Geometry check sheet. Reference: the model listing, model coordinates, mm. A direction names the side the tool comes from. Round coordinates to 2 decimals unless told otherwise and drop trailing zeros. Write each loop counter-clockwise with the first axis right and the second up, starting at its lowest first coordinate (ties: lowest second). Pieces come first, ordered by that corner, then holes. Notation, with made-up numbers: M 70,71.25 L 128,71.25 A31 ccw 128,100.25 Z; hole C 73,16.25 d2. An arc over 180 degrees is marked long. Use a Markdown table: item, result.
```python
from build123d import *

# Parameters (mm, degrees)
F0_W     = 343.231324
F0_H     = 343.231324
F1_DEPTH = 12.7


with BuildPart() as f1:
    # F0 (on Front) → F1 (new body)
    with BuildSketch(Plane.XZ):
        Rectangle(F0_W, F0_H)
        with BuildLine():
            ThreePointArc((-114.373991, 87.598695), (-86.679587, 115.357074), (-57.301, 89.38774))
            Line((-57.301, 89.38774), (-57.223991, -84.985509))
            ThreePointArc((-57.223991, -84.985509), (-84.931642, -113.586746), (-114.373991, -86.774572))
            ThreePointArc((-114.373991, -86.774572), (-114.429209, -84.998141), (-114.373991, -83.22171))
            Line((-114.373991, -83.22171), (-114.373991, 85.938318))
            ThreePointArc((-114.373991, 85.938318), (-114.386042, 86.768506), (-114.373991, 87.598695))
        make_face(mode=Mode.SUBTRACT)
        with BuildLine():
            ThreePointArc((114.411461, 86.554876), (114.417905, 85.362723), (114.374665, 84.171337))
            Line((114.374665, 84.171337), (111.931052, -74.1199))
            ThreePointArc((111.931052, -74.1199), (114.392674, -86.177603), (111.560034, -98.153576))
            ThreePointArc((111.560034, -98.153576), (80.104585, -113.767264), (57.224665, -87.126286))
            ThreePointArc((57.224665, -87.126286), (57.190861, -85.736104), (57.224665, -84.345923))
            Line((57.224665, -84.345923), (57.224665, 85.103969))
            ThreePointArc((57.224665, 85.103969), (57.216092, 85.804222), (57.224665, 86.504474))
            ThreePointArc((57.224665, 86.504474), (85.793493, 114.406821), (114.411461, 86.554876))
        make_face(mode=Mode.SUBTRACT)
    extrude(amount=F1_DEPTH)


solid = f1.part
```
Item 1: Cross-section at A-A, the plane y = -10.5. Record the cut outline in (x, z).
Outcome:
| item | result |
|---|---|
| outline | M -171.62,-171.62 L 171.62,-171.62 L 171.62,171.62 L -171.62,171.62 Z; hole M -114.37,-86.77 A28.6 ccw -57.22,-84.99 L -57.3,89.39 A28.6 ccw -114.37,87.6 A28.6 ccw -114.37,85.94 L -114.37,-83.22 A28.6 ccw Z; hole M 57.22,-87.13 A28.6 ccw 111.56,-98.15 A28.6 ccw 111.93,-74.12 L 114.37,84.17 A28.6 ccw 114.41,86.55 A28.6 ccw 57.22,86.5 A28.6 ccw 57.22,85.1 L 57.22,-84.35 A28.6 ccw Z |
Item 2: Cross-section at D-D, the plane z = -107. Record the cut outline in (x, y), and give its area (3 significant figures).
Outcome:
| item | result |
|---|---|
| outline | M -171.62,-12.7 L -104.1,-12.7 L -104.1,0 L -171.62,0 Z; M -67.55,-12.7 L 66.66,-12.7 L 66.66,0 L -67.55,0 Z; M 104.92,-12.7 L 171.62,-12.7 L 171.62,0 L 104.92,0 Z |
| area | 3,410 mm2 |
Item 3: Access from +Z, -Z, +X, -X, +Y, -Y to the whole of each face (thin tool, end or side, straight path). Record for faces 1 (the face through (-2, -6, -171.616)), 2 (the face through (-114.374, -6, 0)).
Outcome:
| item | result |
|---|---|
| face 1 | -Z, +X, -X, +Y, -Y |
| face 2 | +Y, -Y |
Item 4: Cross-section at C-C, the plane z = 34.5. Record the cut outline in (x, y).
Outcome:
| item | result |
|---|---|
| outline | M -171.62,-12.7 L -114.37,-12.7 L -114.37,0 L -171.62,0 Z; M -57.28,-12.7 L 57.22,-12.7 L 57.22,0 L -57.28,0 Z; M 113.61,-12.7 L 171.62,-12.7 L 171.62,0 L 113.61,0 Z |
Item 5: Cross-section at B-B, the plane x = -80. Record the cut outline in (y, z), and give its area (3 significant figures).
Outcome:
| item | result |
|---|---|
| outline | M -12.7,-171.62 L 0,-171.62 L 0,-113 L -12.7,-113 Z; M -12.7,114.78 L 0,114.78 L 0,171.62 L -12.7,171.62 Z |
| area | 1,470 mm2 |
Item 6: Material ranges on line 1 along X through (y, z) = (-9.5, 88); line 2 along X through (y, z) = (-3.75, -80) (3 decimals); line 3 along Z through (x, y) = (-71.5, -8.25), recorded low to high. Write a range as from..to.
Outcome:
| item | result |
|---|---|
| line 1 | x = -171.62..-114.36, -57.3..57.3, 114.34..171.62 |
| line 2 | x = -171.616..-114.374, -57.226..57.225, 113.815..171.616 |
| line 3 | z = -171.62..-109.75, 111.55..171.62 |
Item 7: Mould release check, pull along X, two halves, no side actions. Record for faces 3 (the face through (-2, 0, 2)), 4 (the face through (171.616, -6, -2)), 5 (the face through (-84.32, -6.26, -113.56)): +X half, -X half, draft (parallel to the pull), parting line (faces both ways), or undercut.
Outcome:
| item | result |
|---|---|
| face 3 | draft |
| face 4 | +X half |
| face 5 | undercut |
